Autodesk Fusion 360 part; units mm, degrees
sketch "Sketch1" plane through (0, 0, 0) normal (0, 1, 0) x (1, 0, 0)
  line L0 (-115, 0) -> (-115, -14.7579)
  line L1 (-110.5022, -35.0449) -> (0, -272)
  arc A0 (-115, -14.7579) -> (-110.5022, -35.0449) centre (-67, -14.7579) ccw
  line L2 (-55, -15) -> (-50, -15)
  line L3 (-24, -132) -> (-50, -76.2428)
  line L4 (-24, -132) -> (-24, -70.4788) construction
  line L5 (-24, -132) -> (-18, -132)
  line L6 (-18, -132) -> (-18, -134)
  line L7 (-18, -134) -> (0, -134)
  line L8 (0, -134) -> (0, -272)
  line L9 (-50, -15) -> (-50, -76.2428)
  line L10 (-55, -2) -> (-57, 0)
  line L11 (-115, 0) -> (-57, 0)
  line L12 (-55, -15) -> (-55, -2)
  point P0 (-115, -25.4)
  dimension "d3" = 25.4
  dimension "d4" = 48
  dimension "d12" = 25
revolve "Revolve2" add sketch "Sketch1" angle 360 about axis through (0, 0, 1.75) along (0, 0, 1)
hole "Hole1" at (0, 0, 134) direction (0, 0, 1) diameter 20 depth 42 tip angle 118
thread "Thread1" thread offset 0 thread length 30
fillet "Fillet3" radius 5 1 edges at (-22.3759, 8.6788, 132)
fillet "Fillet4" radius 10 1 edges at (-46.6164, 18.0808, 76.2428)
fillet "Fillet5" radius 0.8 1 edges at (-51.278, 19.8888, 15)
sketch "Sketch2" plane through (0, 0, 0) normal (0, 0, -1) x (-1, 0, 0)
  circle A0 centre (0, 0) radius 115
  circle A1 centre (0, 0) radius 57
  circle A2 centre (0, 0) radius 80
  circle A3 centre (0, 80) radius 13.25
  point P0 (-47.0228, 64.7214)
  point P1 (-76.0845, 24.7214)
  point P2 (-76.0845, -24.7214)
  point P3 (-47.0228, -64.7214)
  point P4 (0, -80)
  point P5 (47.0228, -64.7214)
  point P6 (76.0845, -24.7214)
  point P7 (76.0845, 24.7214)
  point P8 (47.0228, 64.7214)
  dimension "d31" = 160
  dimension "d32" = 26.5
  dimension "d35" = 360
hole "Hole2" at (0, 80, 0) at (-76.0845, 24.7214, 0) at (-76.0845, -24.7214, 0) at (-47.0228, 64.7214, 0) at (47.0228, 64.7214, 0) at (76.0845, 24.7214, 0) at (76.0845, -24.7214, 0) at (47.0228, -64.7214, 0) at (0, -80, 0) at (-47.0228, -64.7214, 0) direction (0, 0, 1) diameter 26.5 depth 42 tip angle 118
thread "Thread2" thread offset 0 thread length 33
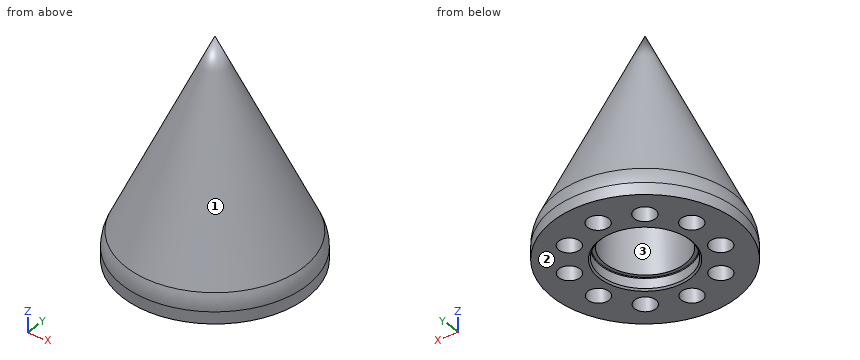
Source: CAD feature listing. Evaluate the final solid. Frame: model axes, mm. Face numbers are marked on the shaded views. Give positions to 0.01 mm unless a question says otherwise; leave off trailing zeros. Write each loop counter-clockwise with the first axis right and the second up, starting at its lowest first coordinate (ties: lowest second). Pieces come first, ordered by that corner, then holes. Notation, with made-up numbers: M -34.5,47.5 L 8.5,47.5 A37 ccw 8.5,84.5 Z; hole C 67,79 d3. An arc over 180 degrees is marked long. Return JSON: item names as keys, results as strings. Group by question number.
1) Pull-direction query (X, two-part tool) for the marked faces 1, 2 and 3; classes: pulls with the +X half, pulls with the -X half, needs draft (parallel to the pull), parting line crosses it, or undercut.
2) Material intervals for line 1 along Y through (x, z) = (0, 29); line 2 along Y through (x, z) = (-51, 22.5); line 3 along Y through (x, z) = (0, 34), sorted ascending. Write a range as [from, to].
3) Pin query (flat end, axial travel): P1, Ø16, axis at x = -76.08, y = 24.72, coming from the -Z side; P2, Ø8, axis at x = 9.5, z = 190, coming from the +Y side; P3, Ø10, axis at x = -64.5, y = 59.5, coming from the +Z side; P4, Ø5, axis at y = -40.5, z = 193.5, coming from the -X side. Return the tip coordinate at first contact, or that it passes through.
4) Cut plane B-B, the plane z = 165. Output: boundary loops of the cut face in (x, y).
5) Cut plane A-A, the plane z = 60. Output: boundary loops of the cut face in (x, y).
Recorded:
{
 "1": {"face 1": "parting line crosses it", "face 2": "needs draft", "face 3": "undercut"},
 "2": {"line 1": "y = [-112.84, -93.25], [-66.75, -50], [50, 66.75], [93.25, 112.84]", "line 2": "y = [-102.37, -77.36], [-52.08, 52.08], [77.36, 102.37]", "line 3": "y = [-110.97, -93.25], [-66.75, -50], [50, 66.75], [93.25, 110.97]"},
 "3": {"P1": "stops at z = 45.15", "P2": "stops at y = 39.16", "P3": "stops at z = 94.55", "P4": "passes through"},
 "4": {"outline": "C 0,0 d99.8; hole C 0,0 d20"},
 "5": {"outline": "C 0,0 d197.73; hole C 0,0 d100"}
}
